Check sheet for the drawn part. Datum: minimum x, y, z corner. Units: mm. Round coordinates to 2 decimals unless told otherwise and drop trailing zeros. Write each loop counter-clockwise with the first axis right and the second up, starting at its lowest first coordinate (ties: lowest second). Pieces come first, ordered by that corner, then holes.
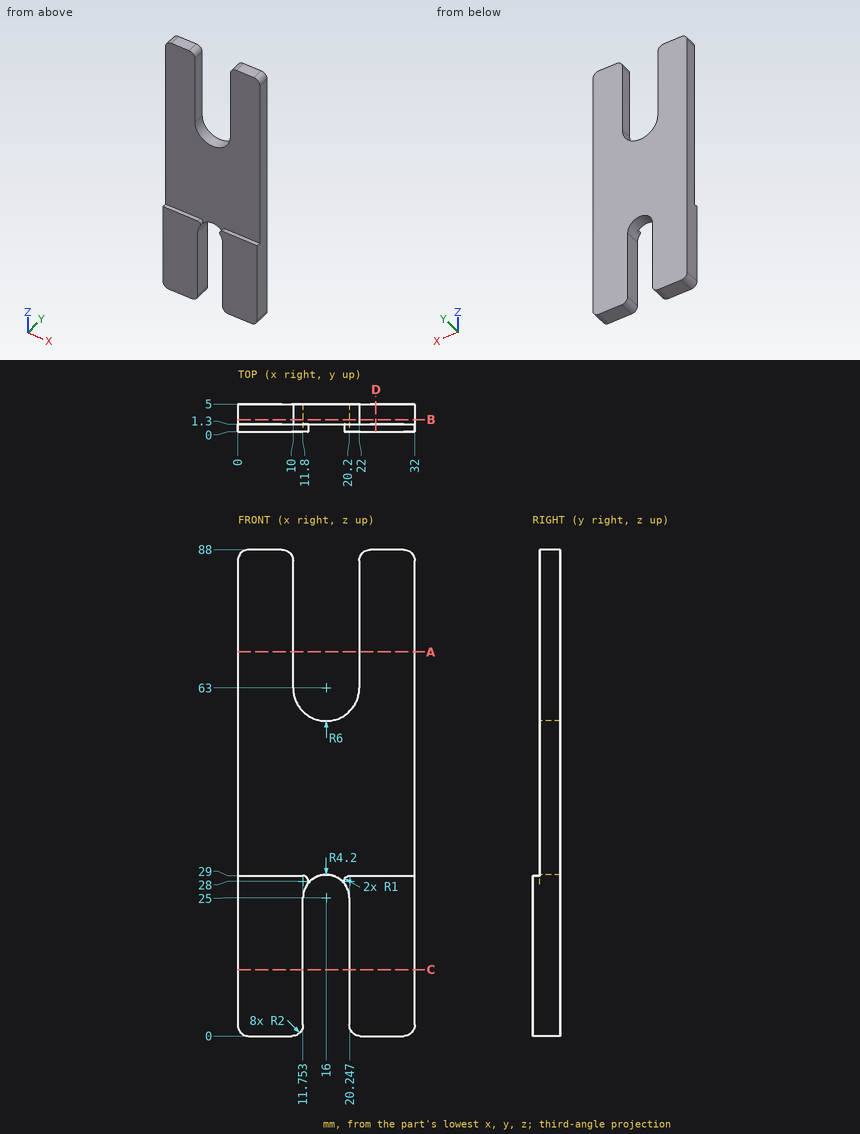
1. Sectioned sample at C-C, the plane z = 12. Enter the section's corners in (x, y), plus the area to 3 significant figures.
2. Sectioned sample at B-B, the plane y = 2.15. Enter the section's corners in (x, z).
3. Scan lines: line 1 along X through (y, z) = (4.35, 79); line 2 along X through (y, z) = (1.85, 22); line 3 along Y through (x, z) = (22.5, 31). Record each from-to range of solid material in increasing order.
4. Sectioned sample at D-D, the plane x = 25. Enter the section's corners in (y, z), plus the area to 3 significant figures.
5. Go/stop test with flat-tipped pins: pin 1 (0.7 mm diameter, centred on x = 5, y = 0.5, fed in from +Z); pin 2 (1.5 mm diameter, centred on x = 20.5, y = 2.5, fed in from -Z); pin 3 (6 mm diameter, centred on x = 10.5, z = 66, fed in from -Y). Record where each tip stops, or that it passes through.
6. Sectioned sample at A-A, the plane z = 69.5. Enter the section's corners in (x, y), plus the area to 3 significant figures.
Computed values:
1. outline: (0, 0) - (11.8, 0) - (11.8, 5) - (0, 5) - close; (20.2, 0) - (32, 0) - (32, 5) - (20.2, 5) - close
1. area: 118 mm2
2. outline: (0, 2) arc R2 ccw to (2, 0) - (9.8, 0) arc R2 ccw to (11.8, 2) - (11.8, 25) arc R4.2 cw to (20.2, 25) - (20.2, 2) arc R2 ccw to (22.2, 0) - (30, 0) arc R2 ccw to (32, 2) - (32, 86) arc R2 ccw to (30, 88) - (24, 88) arc R2 ccw to (22, 86) - (22, 63) arc R6 cw to (10, 63) - (10, 86) arc R2 ccw to (8, 88) - (2, 88) arc R2 ccw to (0, 86) - close
3. line 1: x = 0 to 10, 22 to 32
3. line 2: x = 0 to 11.8, 20.2 to 32
3. line 3: y = 1.3 to 5
4. outline: (0, 0) - (5, 0) - (5, 88) - (1.3, 88) - (1.3, 29) - (0, 29) - close
4. area: 363 mm2
5. pin 1: stops at z = 29
5. pin 2: stops at z = 0.24
5. pin 3: stops at y = 1.3
6. outline: (0, 1.3) - (10, 1.3) - (10, 5) - (0, 5) - close; (22, 1.3) - (32, 1.3) - (32, 5) - (22, 5) - close
6. area: 74.0 mm2
